```python
from build123d import *

# Parameters (mm, degrees)
F0_R      = 3
F0_R_2    = 10.5
F1_DEPTH  = 42
F2_R      = 3
F3_DEPTH  = 21
F4_R      = 16
F5_DEPTH  = 85
F6_SIZE   = 2
F7_R      = 2
F8_DEPTH  = 25
F9_R      = 2
F10_DEPTH = 25


with BuildPart() as f1:
    # F0 (on Right) → F1 (new body)
    with BuildSketch(Plane.YZ):
        Polygon((70.5, -116.2), (112.5, -116.2), (112.5, -74.2), (-70.5, 116.2), (-112.5, 116.2), (-112.5, 74.2), align=None)
        with Locations((-10, -10)):
            Circle(F0_R, mode=Mode.SUBTRACT)
        with Locations((10, -10)):
            Circle(F0_R, mode=Mode.SUBTRACT)
        with Locations((-10, 10)):
            Circle(F0_R, mode=Mode.SUBTRACT)
        with Locations((-91.5, 95.2)):
            Circle(F0_R_2, mode=Mode.SUBTRACT)
        with Locations((10, 10)):
            Circle(F0_R, mode=Mode.SUBTRACT)
    extrude(amount=F1_DEPTH)

    # F2 (on face) → F3 (cut)
    with BuildSketch(Plane.YZ.offset(42)):
        Polygon((12.831933, -56.2), (95.19958, -56.2), (-12.831933, 56.2), (-95.19958, 56.2), align=None)
        with Locations((-10, -10)):
            Circle(F2_R, mode=Mode.SUBTRACT)
        with Locations((10, -10)):
            Circle(F2_R, mode=Mode.SUBTRACT)
        with Locations((-10, 10)):
            Circle(F2_R, mode=Mode.SUBTRACT)
        with Locations((10, 10)):
            Circle(F2_R, mode=Mode.SUBTRACT)
    extrude(amount=-F3_DEPTH, mode=Mode.SUBTRACT)

    # F4 (on face) → F5 (cut)
    with BuildSketch(Plane(origin=(0, 112.5, 0), x_dir=(-1, 0, 0), z_dir=(0, 1, 0))):
        with Locations((-21, -95.2)):
            Circle(F4_R)
    extrude(amount=-F5_DEPTH, mode=Mode.SUBTRACT)

    # F6
    f6_edges = [f1.edges().sort_by_distance(p)[0] for p in [
        (21, 41.183824, 0),
        (21, -41.183824, 0),
        (42, -54.015756, 56.2),
        (0, -91.5, 116.2),
        (0, 91.5, -116.2),
        (42, 54.015756, -56.2),
        (42, 91.5, -116.2),
        (42, -91.5, 116.2),
    ]]
    chamfer(f6_edges, length=F6_SIZE)

    # F7 (on face) → F8 (cut)
    with BuildSketch(Plane.XY.offset(116.2)):
        with Locations((21, -91.5)):
            Circle(F7_R)
    extrude(amount=-F8_DEPTH, mode=Mode.SUBTRACT)

    # F9 (on face) → F10 (cut)
    with BuildSketch(Plane(origin=(0, 0, -116.2), x_dir=(1, 0, 0), z_dir=(0, 0, -1))):
        with Locations((21, -91.5)):
            Circle(F9_R)
    extrude(amount=-F10_DEPTH, mode=Mode.SUBTRACT)


solid = f1.part
```
CAD build for the part. Positions are in the model's coordinates, mm. A direction names the side the tool comes from. Coordinates: 2 decimals unless noted, no trailing zeros. Write each loop counter-clockwise with the first axis right and the second up, starting at its lowest first coordinate (ties: lowest second). Pieces come first, ordered by that corner, then holes. Notation, with made-up numbers: (-31, 4.25) -> (-26, 4.25) arc R25 cw to (-26, 30.25) -> close; hole circle Ø7 at (18.25, 45.25). An arc over 180 degrees is marked (long way). Use CSV: the item, a comma, the result in double quotes. Start each with the question number.
Item 1: Two-plate mould, pull along Y, no slides. Class faces 3 (the cylindrical face through (10.35, -12.21, -7.97)), 4 (the flat face through (42, 74, -80)), 5 (the flat face through (16.04, 22.28, 19.67)), 6 (the cylindrical face through (10.35, 12.77, 8.85)): +Y half, -Y half, draft (parallel to the pull), parting line (faces both ways), or undercut.
Item 2: Band-saw the part on A-A, the plane x = 8. Write the cut outline in (y, z).
Item 3: Band-saw the part on D-D, the plane x = 26.5. Write the cut outline in (y, z), plus the area to 3 significant figures.
Item 4: Tool access for faces 1 (the flat face through (25, -91, 116.2)), 2 (the flat face through (21, -1, 1)): list every direction of +Z, -Z, +X, -X, +Y, -Y with a clear straight run to the whole face (end or side of a thin tool).
Item 5: Wall check: probe 1 along X at (y, z) = (91, -114); probe 2 along Z at (x, y) = (10, -10); probe 3 along X at (y, z) = (25, -14). Give the ranges that are in metal, low to high.
Item 6: Drop flat-ended pins along their axis: P1, Ø23, axis at x = 25, y = -64.5, coming from the -Z side; P2, Ø6, axis at x = 11, z = -33.5, coming from the +Y side; P3, Ø17, axis at x = 34.5, y = 71.5, coming from the +Z side. Give the stop position or say it passes through.
Item 7: Band-saw the part on C-C, the plane y = -10. Write the cut outline in (x, z), plus the area to 3 significant figures.
Item 8: Band-saw the part on B-B, the plane z = -95.2. Write the cut outline in (x, y), plus the area to 3 significant figures.
Response values:
1,face 3,"undercut"
1,face 4,"draft"
1,face 5,"+Y half"
1,face 6,"undercut"
2,outline,"(-112.5, 74.2) -> (41.35, -85.87) -> (112.5, -85.87) -> (112.5, -74.2) -> (-70.5, 116.2) -> (-112.5, 116.2) -> close; (59.28, -104.53) -> (70.5, -116.2) -> (112.5, -116.2) -> (112.5, -104.53) -> close; hole circle Ø21 at (-91.5, 95.2); hole circle Ø6 at (-10, -10); hole circle Ø6 at (-10, 10); hole circle Ø6 at (10, -10); hole circle Ø6 at (10, 10)"
3,outline,"(-112.5, 74.2) -> (-95.2, 56.2) -> (-12.83, 56.2) -> (-70.5, 116.2) -> (-112.5, 116.2) -> close; (12.83, -56.2) -> (35.88, -80.18) -> (112.5, -80.18) -> (112.5, -74.2) -> (95.2, -56.2) -> close; (64.76, -110.22) -> (70.5, -116.2) -> (112.5, -116.2) -> (112.5, -110.22) -> close; hole circle Ø21 at (-91.5, 95.2)"
3,area,"5,970 mm2"
4,face 1,"+Z, +X, -X, +Y, -Y"
4,face 2,"+X, +Y, -Y"
5,probe 1,"x = 0 to 19.06, 22.94 to 42"
5,probe 2,"z = -32.44 to -13, -7 to 7, 13 to 53.25"
5,probe 3,"x = 0 to 21"
6,P1,"stops at z = 14.05"
6,P2,"stops at y = 76.27"
6,P3,"stops at z = -56.2"
7,outline,"(0, -32.44) -> (19, -32.44) -> (21, -29.56) -> (21, -13) -> (0, -13) -> close; (0, -7) -> (21, -7) -> (21, 7) -> (0, 7) -> close; (0, 13) -> (21, 13) -> (21, 50.37) -> (19, 53.25) -> (0, 53.25) -> close"
7,area,"1,540 mm2"
8,outline,"(0, 50.32) -> (5, 50.32) -> (5, 112.5) -> (0, 112.5) -> close; (37, 50.32) -> (42, 50.32) -> (42, 112.5) -> (37, 112.5) -> close"
8,area,"622 mm2"
